Here's how the part is built. I have some questions about the finished solid (model axes, mm). Give positions to 0.01 mm unless a question says otherwise; leave off trailing zeros. Write each loop counter-clockwise with the first axis right and the second up, starting at its lowest first coordinate (ties: lowest second). Pieces come first, ordered by that corner, then holes. Notation, with made-up numbers: (5, 26.25) - (35, 26.25) arc R23 cw to (35, 43.25) - close; hole circle Ø5 at (14.25, 82.25). An arc over 180 degrees is marked (long way). Write each question's results on one line, items separated by ' | '. Start each with the question number.
Item 1: Suppose I cut it at C-C on y = 46. List the corners of the cut face in (x, z) for me, then the cut area to 3 significant figures.
Item 2: Suppose I cut it at A-A on z = 0.15. List the corners of the cut face in (x, y) for me, then the cut area to 3 significant figures.
Item 3: Suppose I cut it at B-B on x = 21. List the corners of the cut face in (y, z) for me, then the cut area to 3 significant figures.
Item 4: Please list where these lines run through material, in increasing order: line 1 along Y through (x, z) = (-20, 0.35); line 2 along Y through (x, z) = (-2.5, 0.6); line 3 along X through (y, z) = (45, 0.65).
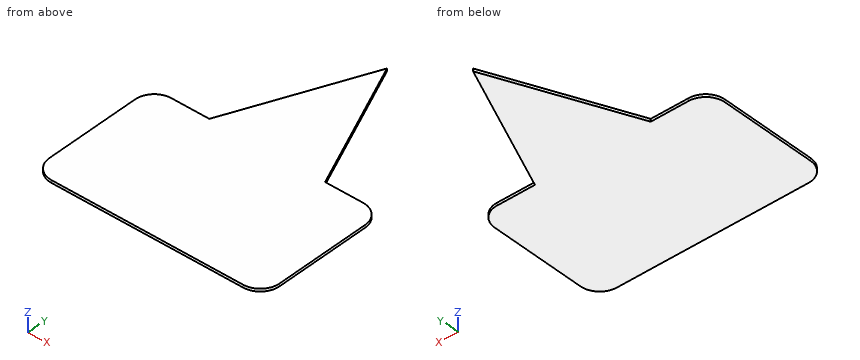
```python
from build123d import *

# Parameters (mm, degrees)
F1_DEPTH = 0.7


with BuildPart() as f1:
    # F0 (on Top) → F1 (new body)
    with BuildSketch(Plane.XY):
        with BuildLine():
            Line((-25, 0), (0, 0))
            Line((0, 0), (25, 0))
            ThreePointArc((25, 0), (28.535534, 1.464466), (30, 5))
            Line((30, 5), (30, 30))
            ThreePointArc((30, 30), (28.535534, 33.535534), (25, 35))
            Line((25, 35), (15.099166, 35))
            Line((15.099166, 35), (0, 70))
            Line((0, 70), (-15.099166, 35))
            Line((-15.099166, 35), (-25, 35))
            ThreePointArc((-25, 35), (-28.535534, 33.535534), (-30, 30))
            Line((-30, 30), (-30, 5))
            ThreePointArc((-30, 5), (-28.535534, 1.464466), (-25, 0))
        make_face()
    extrude(amount=F1_DEPTH)


solid = f1.part
```
Checked values:
1) outline: (-10.35, 0) - (10.35, 0) - (10.35, 0.7) - (-10.35, 0.7) - close | area: 14.5 mm^2
2) outline: (-30, 5) arc R5 ccw to (-25, 0) - (25, 0) arc R5 ccw to (30, 5) - (30, 30) arc R5 ccw to (25, 35) - (15.1, 35) - (0, 70) - (-15.1, 35) - (-25, 35) arc R5 ccw to (-30, 30) - close | area: 2,610 mm^2
3) outline: (0, 0) - (35, 0) - (35, 0.7) - (0, 0.7) - close | area: 24.5 mm^2
4) line 1: y = 0 to 35 | line 2: y = 0 to 64.2 | line 3: x = -10.79 to 10.79
